Geometry: final body of the model. Coordinates: model frame, mm. A direction names the side the tool comes from. Give positions to 0.01 mm unless a question says otherwise; leave off trailing zeros. Loops run counter-clockwise (first coordinate to the right, second up) from the corner with the lowest first, then second, coordinate; pieces in that order, holes last. Notation, with made-up numbers: (9.25, -23.5) -> (59.25, -23.5) arc R21 cw to (59.25, 14.5) -> close; hole circle Ø9 at (80, 40). An arc over 180 degrees is marked (long way). One line per question, with ' | ' between items. Start each with the question number.
Item 1: Material intervals for line 1 along Z through (x, y) = (-3.5, 3); line 2 along X through (y, z) = (-2, 1.25); line 3 along Y through (x, z) = (0, -2), sorted ascending. Write a range as [from, to].
Item 2: Section A-A on z = 0.5. Return loops of the section in (x, y).
Item 3: Mould query, pull axis X, two halves, no side actions, for faces 1 (the flat face through (1.8, 3, 1.2)), 2 (the conical face through (0.08, -3.652, 2.412)), 3 (the flat face through (-1.726, 3.045, 1.232)), 4 (the flat face through (2, -2, -0.5)). Classes: released by +X, released by -X, zero draft, split by the parting line, or undercut.
Item 4: Pin query (flat end, axial travel): P1, Ø6, axis at y = -1, z = -8.5, coming from the -X side; P2, Ø1.5, axis at x = 1.5, z = -7.5, coming from the -Y side; P3, Ø6, axis at y = -3.5, z = -2.5, coming from the +X side. Return the tip coordinate at first contact, or that it passes through.
Item 5: Set-up query: faces 5 (the flat face through (1.726, -3.045, 1.232)), 6 (the flat face through (3, -3, 0)), 7 (the flat face through (-3.5, 0, 1)). Return all of +Z, -Z, +X, -X, +Y, -Y with unobstructed straight access to the full face (end or side cutting, diameter ignored); none if empty.
Item 6: Section C-C on z = -9.5. Return loops of the section in (x, y), then the cut area to 3 significant figures.
Item 7: Section B-B on y = 4.25. Return loops of the section in (x, z).
Solid Edge part; units mm, degrees
sketch "Sketch1" plane through (0, 0, 0) normal (0, -1, 0) x (1, 0, 0)
  line L0 (2.5, -0.5) -> (2.5, -10.5)
  line L1 (2.5, -10.5) -> (0, -10.5)
  line L2 (0, -10.5) -> (0, 0)
  line L3 (0, 0) -> (5, 0)
  line L4 (5, 0) -> (5, -0.5)
  line L5 (5, -0.5) -> (2.5, -0.5)
revolve "RevolvedProtrusion1" add sketch "Sketch1" angle 360 about axis through (0, 0, -10.5) along (0, 0, 1)
sketch "Sketch2" plane through (0, 0, 0) normal (0, 0, 1) x (-1, 0, 0)
  line L0 (3.5, -2.0207) -> (3.5, 2.0207)
  line L1 (3.5, 2.0207) -> (0, 4.0415)
  line L2 (0, 4.0415) -> (-3.5, 2.0207)
  line L3 (-3.5, 2.0207) -> (-3.5, -2.0207)
  line L4 (-3.5, -2.0207) -> (0, -4.0415)
  line L5 (0, -4.0415) -> (3.5, -2.0207)
extrude "Protrusion1" add sketch "Sketch2" along normal blind 2.5
sketch "Sketch3" plane through (0, 0, 0) normal (0, -1, 0) x (1, 0, 0)
  line L0 (6.0981, 2.5) -> (3.5, 2.5)
  line L1 (3.5, 2.5) -> (6.0981, 1)
  line L2 (6.0981, 1) -> (6.0981, 2.5)
revolve "RevolvedCutout1" cut sketch "Sketch3" angle 360 about axis through (0, 0, 3.8117) along (0, 0, -1)
Result sheet:
1) line 1: z = [-0.5, 0] | line 2: x = [-3.5, 3.5] | line 3: y = [-2.5, 2.5]
2) outline: (-3.5, -2.02) -> (0, -4.04) -> (3.5, -2.02) -> (3.5, 2.02) -> (0, 4.04) -> (-3.5, 2.02) -> close
3) face 1: released by +X | face 2: split by the parting line | face 3: released by -X | face 4: zero draft
4) P1: stops at x = -2.5 | P2: stops at y = -2.38 | P3: stops at x = 4.84
5) face 5: +Z, +X, -Y | face 6: +Z | face 7: +Z, -X, +Y, -Y
6) outline: circle Ø5 at (0, 0) | area: 19.6 mm²
7) outline: (-2.63, -0.5) -> (2.63, -0.5) -> (2.63, 0) -> (-2.63, 0) -> close
